Drawing for the job (mm, zero at the part's lowest x, y, z). Give positions to 0.01 mm unless a question says otherwise; leave off trailing zeros. Order: outer loops, then holes, each group sorted by start corner. A loop starts at its lowest first (then second) coordinate and runs counter-clockwise, first axis right, second up. Notation, with made-up numbers: (55, 20) - (102, 20) arc R25 cw to (102, 42) - close; hole circle Ø2 at (-6, -12.5). An arc over 180 degrees is marked (long way). One line per item, written item: value.
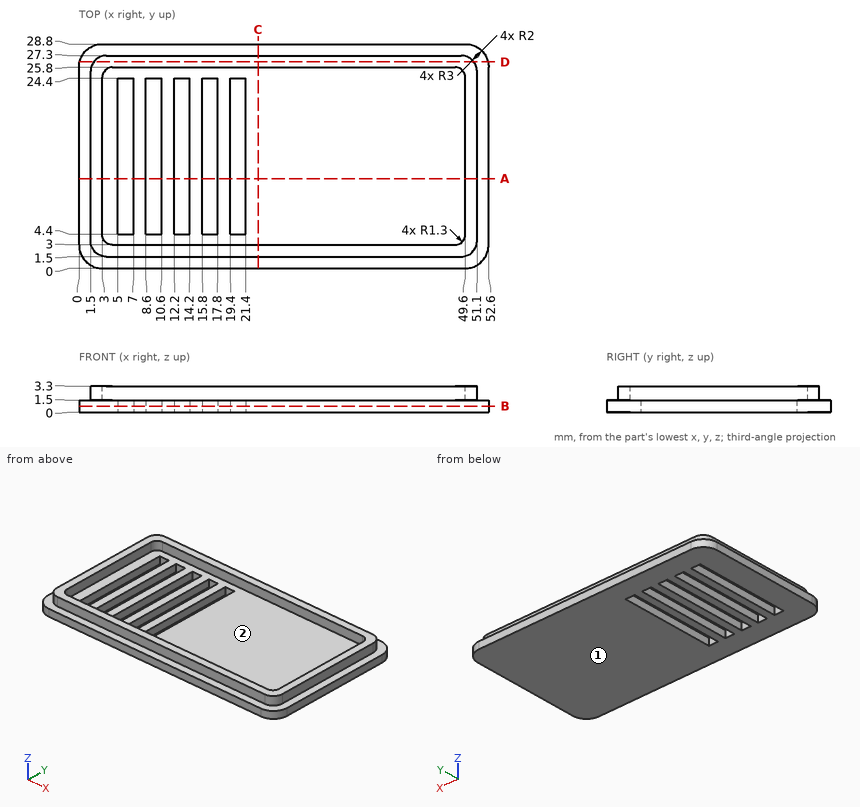
1) Cut at D-D, the plane y = 26.5. Give the cut face in (x, z).
Outcome:
outline: (0.08, 0) - (52.52, 0) - (52.52, 1.5) - (50.7, 1.5) - (50.7, 3.3) - (1.9, 3.3) - (1.9, 1.5) - (0.08, 1.5) - close
2) Mould opens along Y. For the marked faces 1 and 2 say: released by +Y, released by -Y, zero draft, split by the parting line, or undercut.
Outcome:
face 1: zero draft
face 2: undercut
3) Pin check, flat tips, straight feed: pin 1 (7 mm diameter, centred on x = 29.5, y = 14, fed in from +Z); pin 2 (10 mm diameter, centred on x = 17, y = 6.5, fed in from +Z). Stop position of each tip, or through.
Outcome:
pin 1: stops at z = 1.5
pin 2: stops at z = 3.3
4) Cut at C-C, the plane x = 23. Give the cut face in (y, z).
Outcome:
outline: (0, 0) - (28.8, 0) - (28.8, 1.5) - (27.3, 1.5) - (27.3, 3.3) - (25.8, 3.3) - (25.8, 1.5) - (3, 1.5) - (3, 3.3) - (1.5, 3.3) - (1.5, 1.5) - (0, 1.5) - close
5) Drill centre lines: line 1 along X through (y, z) = (18.5, 0.55); line 2 along X through (y, z) = (21.25, 2.65); line 3 along Y through (x, z) = (18, 2.5). Where is each one in solid material? Low to high. Write a range as from..to.
Outcome:
line 1: x = 0..5, 7..8.6, 10.6..12.2, 14.2..15.8, 17.8..19.4, 21.4..52.6
line 2: x = 1.5..3, 49.6..51.1
line 3: y = 1.5..3, 25.8..27.3
6) Cut at B-B, the plane z = 0.75. Give the cut face in (x, y), then the cut area to 3 significant figures.
Outcome:
outline: (0, 3) arc R3 ccw to (3, 0) - (49.6, 0) arc R3 ccw to (52.6, 3) - (52.6, 25.8) arc R3 ccw to (49.6, 28.8) - (3, 28.8) arc R3 ccw to (0, 25.8) - close; hole (5, 4.4) - (7, 4.4) - (7, 24.4) - (5, 24.4) - close; hole (8.6, 4.4) - (10.6, 4.4) - (10.6, 24.4) - (8.6, 24.4) - close; hole (12.2, 4.4) - (14.2, 4.4) - (14.2, 24.4) - (12.2, 24.4) - close; hole (15.8, 4.4) - (17.8, 4.4) - (17.8, 24.4) - (15.8, 24.4) - close; hole (19.4, 4.4) - (21.4, 4.4) - (21.4, 24.4) - (19.4, 24.4) - close
area: 1,310 mm^2
7) Cut at A-A, the plane y = 11.5. Give the number of separate pieces and of enclosed holes in the cut face, then the cut area to 3 significant figures.
Outcome:
separate pieces: 6
enclosed holes: 0
area: 69.3 mm^2
